from build123d import *

# Parameters (mm, degrees)
SKETCH1_R                       = 26
SKETCH1_R_2                     = 20
RELIEVED_FLOATING_RING_DEPTH    = 4
SKETCH2_W                       = 20
SKETCH2_H                       = 8
X_SLIDE_PAD_1_DEPTH             = 4
SKETCH3_W                       = 8
SKETCH3_H                       = 20
Y_SLIDE_PAD_1_DEPTH             = 4
SKETCH4_W                       = 20
SKETCH4_H                       = 8
X_SLIDE_PAD_1_2_DEPTH           = 4
SKETCH5_W                       = 8
SKETCH5_H                       = 20
Y_SLIDE_PAD_1_2_DEPTH           = 4
SKETCH6_W                       = 4.1
SKETCH6_H                       = 90
LOWER_Y_SLOTS_W4P1_H2_DEPTH     = 2
SKETCH7_W                       = 90
SKETCH7_H                       = 4.1
UPPER_X_SLOTS_W4P1_H2_DEPTH     = 2
BENCH_UPPERX_W4P030_1_1_START   = 2
SKETCH8_W                       = 20
SKETCH8_H                       = 0.045
BENCH_UPPERX_W4P030_1_1_DEPTH   = 2
SKETCH9_W                       = 20
SKETCH9_H                       = 0.045
BENCH_UPPERX_W4P030_1_1_2_DEPTH = 2
SKETCH10_W                      = 20
SKETCH10_H                      = 0.045
BENCH_UPPERX_W4P030_1_1_3_DEPTH = 2
SKETCH11_W                      = 20
SKETCH11_H                      = 0.045
BENCH_UPPERX_W4P030_1_1_4_DEPTH = 2
SKETCH12_W                      = 0.045
SKETCH12_H                      = 20
BENCH_LOWERY_W4P030_1_1_DEPTH   = 2
SKETCH13_W                      = 0.045
SKETCH13_H                      = 20
BENCH_LOWERY_W4P030_1_1_2_DEPTH = 2
SKETCH14_W                      = 0.045
SKETCH14_H                      = 20
BENCH_LOWERY_W4P030_1_1_3_DEPTH = 2
SKETCH15_W                      = 0.045
SKETCH15_H                      = 20
BENCH_LOWERY_W4P030_1_1_4_DEPTH = 2


with BuildPart() as part:
    # Sketch1 → Relieved_Floating_Ring (new body)
    with BuildSketch(Plane.XY):
        Circle(SKETCH1_R)
        Circle(SKETCH1_R_2, mode=Mode.SUBTRACT)
    extrude(amount=RELIEVED_FLOATING_RING_DEPTH)

    # Sketch2 → X_Slide_Pad_-1 (add)
    with BuildSketch(Plane.XY):
        with Locations((-34, 0)):
            Rectangle(SKETCH2_W, SKETCH2_H)
    extrude(amount=X_SLIDE_PAD_1_DEPTH)

    # Sketch3 → Y_Slide_Pad_-1 (add)
    with BuildSketch(Plane.XY):
        with Locations((0, -34)):
            Rectangle(SKETCH3_W, SKETCH3_H)
    extrude(amount=Y_SLIDE_PAD_1_DEPTH)

    # Sketch4 → X_Slide_Pad_1 2 (add)
    with BuildSketch(Plane.XY):
        with Locations((34, 0)):
            Rectangle(SKETCH4_W, SKETCH4_H)
    extrude(amount=X_SLIDE_PAD_1_2_DEPTH)

    # Sketch5 → Y_Slide_Pad_1 2 (add)
    with BuildSketch(Plane.XY):
        with Locations((0, 34)):
            Rectangle(SKETCH5_W, SKETCH5_H)
    extrude(amount=Y_SLIDE_PAD_1_2_DEPTH)

    # Sketch6 → Lower_Y_Slots_W4p1_H2 (cut)
    with BuildSketch(Plane(origin=(0, 0, 0), x_dir=(-1, 0, 0), z_dir=(0, 0, -1))):
        Rectangle(SKETCH6_W, SKETCH6_H)
    extrude(amount=-LOWER_Y_SLOTS_W4P1_H2_DEPTH, mode=Mode.SUBTRACT)

    # Sketch7 → Upper_X_Slots_W4p1_H2 (cut)
    with BuildSketch(Plane.XY.offset(4)):
        Rectangle(SKETCH7_W, SKETCH7_H)
    extrude(amount=-UPPER_X_SLOTS_W4P1_H2_DEPTH, mode=Mode.SUBTRACT)

    # Sketch8 → Bench_UpperX_W4p030_-1_-1 (add)
    with BuildSketch(Plane.XY.offset(BENCH_UPPERX_W4P030_1_1_START)):
        with Locations((-34, -2.0375)):
            Rectangle(SKETCH8_W, SKETCH8_H)
    extrude(amount=BENCH_UPPERX_W4P030_1_1_DEPTH)

    # Sketch9 → Bench_UpperX_W4p030_-1_1 2 (add)
    with BuildSketch(Plane.XY.offset(BENCH_UPPERX_W4P030_1_1_START)):
        with Locations((-34, 2.0375)):
            Rectangle(SKETCH9_W, SKETCH9_H)
    extrude(amount=BENCH_UPPERX_W4P030_1_1_2_DEPTH)

    # Sketch10 → Bench_UpperX_W4p030_1_-1 3 (add)
    with BuildSketch(Plane.XY.offset(BENCH_UPPERX_W4P030_1_1_START)):
        with Locations((34, -2.0375)):
            Rectangle(SKETCH10_W, SKETCH10_H)
    extrude(amount=BENCH_UPPERX_W4P030_1_1_3_DEPTH)

    # Sketch11 → Bench_UpperX_W4p030_1_1 4 (add)
    with BuildSketch(Plane.XY.offset(BENCH_UPPERX_W4P030_1_1_START)):
        with Locations((34, 2.0375)):
            Rectangle(SKETCH11_W, SKETCH11_H)
    extrude(amount=BENCH_UPPERX_W4P030_1_1_4_DEPTH)

    # Sketch12 → Bench_LowerY_W4p030_-1_-1 (add)
    with BuildSketch(Plane.XY):
        with Locations((-2.0375, -34)):
            Rectangle(SKETCH12_W, SKETCH12_H)
    extrude(amount=BENCH_LOWERY_W4P030_1_1_DEPTH)

    # Sketch13 → Bench_LowerY_W4p030_-1_1 2 (add)
    with BuildSketch(Plane.XY):
        with Locations((2.0375, -34)):
            Rectangle(SKETCH13_W, SKETCH13_H)
    extrude(amount=BENCH_LOWERY_W4P030_1_1_2_DEPTH)

    # Sketch14 → Bench_LowerY_W4p030_1_-1 3 (add)
    with BuildSketch(Plane.XY):
        with Locations((-2.0375, 34)):
            Rectangle(SKETCH14_W, SKETCH14_H)
    extrude(amount=BENCH_LOWERY_W4P030_1_1_3_DEPTH)

    # Sketch15 → Bench_LowerY_W4p030_1_1 4 (add)
    with BuildSketch(Plane.XY):
        with Locations((2.0375, 34)):
            Rectangle(SKETCH15_W, SKETCH15_H)
    extrude(amount=BENCH_LOWERY_W4P030_1_1_4_DEPTH)


solid = part.part
CAD build for the part. Positions are in the model's coordinates, mm. A direction names the side the tool comes from. Give positions to 0.01 mm unless a question says otherwise; leave off trailing zeros. Write each loop counter-clockwise with the first axis right and the second up, starting at its lowest first coordinate (ties: lowest second). Pieces come first, ordered by that corner, then holes. Notation, with made-up numbers: M 78.25,-9.5 L 119.25,-9.5 A14 ccw 119.25,-4.5 Z; hole C 14,-18.5 d2. An arc over 180 degrees is marked long. Put each result on its own line as item: value. Start each with the question number.
(1) Mould opens along Y. For faces 4 (the face through (18.55, 18.22, 1.97)), 5 (the face through (34, -2.015, 3)), 6 (the face through (-3, -20, 4)) say: +Y half, -Y half, draft (parallel to the pull), parting line (faces both ways), or undercut.
(2) Flat gauge pins, fed straight in: pin 1 Ø2 at (x, z) = (21.5, 2.5) entering from +Y; pin 2 Ø1 at (y, z) = (-10, 1.5) entering from -X; pin 3 Ø1.5 at (y, z) = (-22, 1) entering from +X; pin 4 Ø24 at (x, y) = (0, 0) entering from -Z. Where does each tip first touch, or does it go through?
(3) Band-saw the part on D-D, the plane y = 32. Write the cut outline in (x, z) (3 decimals), and give its area (3 significant figures).
(4) Band-saw the part on A-A, the plane x = 0. Write the cut outline in (y, z).
(5) Which spindle directions (+Z, -Z, +X, -X, +Y, -Y) get a long thin tool onto all of the face, cutting with end or side? Do faces 1 (the face through (4, -35, 2)), 2 (the face through (-35, -4, 2)), 3 (the face through (-34, -2.015, 3)). Say none if no direction does.
(6) Probe L1, parallel to Y at x = 0, z = 2.1; L2, parallel to X at y = 28, z = 1.65 (3 decimals). List the from-to ranges inside material, lowest first.
(7) Band-saw the part on B-B, the plane y = 0. Write the cut outline in (x, z), and give its area (3 significant figures).
Response values:
1. face 4: +Y half
1. face 5: undercut
1. face 6: draft
2. pin 1: stops at y = 15.99
2. pin 2: stops at x = -24.2
2. pin 3: stops at x = 14.98
2. pin 4: passes through
3. outline: M -4,0 L -2.015,0 L -2.015,2 L 2.015,2 L 2.015,0 L 4,0 L 4,4 L -4,4 Z
3. area: 23.9 mm2
4. outline: M -44,2 L -20,2 L -20,4 L -44,4 Z; M 20,2 L 44,2 L 44,4 L 20,4 Z
5. face 1: +Z, -Z, +X, -Y
5. face 2: +Z, -Z, -X, -Y
5. face 3: +Z, +X, -X
6. L1: y = -44 to -20, 20 to 44
6. L2: x = -4 to -2.015, 2.015 to 4
7. outline: M -44,0 L -20,0 L -20,2 L -44,2 Z; M 20,0 L 44,0 L 44,2 L 20,2 Z
7. area: 96.0 mm2
